Autodesk Fusion 360 part; units mm, degrees
sketch "Sketch1" plane through (0, 0, 0) normal (0, 0, 1) x (1, 0, 0)
  line L0 (75, -95) -> (-75, -95)
  line L1 (-75, -95) -> (-75, 95)
  line L2 (-75, 95) -> (75, 95)
  line L3 (75, 95) -> (75, -95)
  line L4 (75, -95) -> (-75, 95) construction
  line L5 (-75, -95) -> (75, 95) construction
  dimension "d1" = 150
  dimension "d2" = 190
ref_plane "WorkPlane1" through (0, 0, 45) normal (0, 0, 1) x (1, 0, 0)
sketch "Sketch2" plane through (0, 0, 45) normal (0, 0, 1) x (1, 0, 0)
  line L0 (75, -95) -> (-75, -95)
  line L1 (-75, -95) -> (-75, 95)
  line L2 (-75, 95) -> (75, 95)
  line L3 (75, 95) -> (75, -95)
  line L4 (75, -95) -> (-75, 95) construction
  line L5 (-75, -95) -> (75, 95) construction
  dimension "d4" = 150
  dimension "d5" = 190
sketch "Sketch3" plane through (0, 0, 45) normal (0, 0, 1) x (1, 0, 0)
ref_plane "WorkPlane2" through (75, 95, 45) normal (-1, 0, 0) x (0, -1, 0)
sketch "Sketch4" plane through (75, 95, 45) normal (-1, 0, 0) x (0, -1, 0)
  circle A0 centre (155, -22.5) radius 50
  line L0 (0, 0) -> (190, 0)
  circle A1 centre (35, -22.5) radius 50
  dimension "d6" = 100
  dimension "d7" = 22.5
  dimension "d8" = 100
  dimension "d9" = 22.5
  dimension "d10" = 120
  dimension "d11" = 155
ref_plane "WorkPlane3" through (-75, -95, 45) normal (1, 0, 0) x (0, 1, 0)
sketch "Sketch5" plane through (-75, -95, 45) normal (1, 0, 0) x (0, 1, 0)
  circle A0 centre (155, -22.5) radius 50
  circle A1 centre (35, -22.5) radius 50
  line L0 (0, 0) -> (190, 0)
  dimension "d12" = 100
  dimension "d13" = 100
  dimension "d14" = 120
  dimension "d15" = 155
  dimension "d16" = 22.5
  dimension "d17" = 22.5
extrude "Extrude1" add sketch "Sketch2" against normal blind 3 makes body 1
extrude "Extrude2" add sketch "Sketch1" along normal blind 3 separate body makes body 2
extrude "Extrude3" add sketch "Sketch4" against normal blind 40 bodies 1 2
extrude "Extrude4" add sketch "Sketch5" against normal blind 40 bodies 1
sketch "Sketch6" plane through (115, 0, 0) normal (1, 0, 0) x (0, 1, 0)
  circle A0 centre (-60, 22.5) radius 50
  circle A1 centre (-60, 22.5) radius 40
  dimension "d26" = -10
sketch "Sketch7" plane through (115, 0, 0) normal (1, 0, 0) x (0, 1, 0)
  circle A0 centre (60, 22.5) radius 50
  circle A1 centre (60, 22.5) radius 40
  dimension "d27" = -10
extrude "Extrude5" cut sketch "Sketch6" sketch "Sketch7" against normal blind 30 contours A1 of sketch 2 contours A1 bodies 1
sketch "Sketch8" plane through (-115, 0, 0) normal (-1, 0, 0) x (0, -1, 0)
  circle A0 centre (-60, 22.5) radius 50
  circle A1 centre (-60, 22.5) radius 40
  dimension "d30" = -10
sketch "Sketch9" plane through (-115, 0, 0) normal (-1, 0, 0) x (0, -1, 0)
  circle A0 centre (60, 22.5) radius 50
  circle A1 centre (60, 22.5) radius 40
  dimension "d31" = -10
extrude "Extrude6" cut sketch "Sketch8" sketch "Sketch9" against normal blind 30 contours A1 of sketch 2 contours A1 bodies 1
CAD build for the part. Positions are in the model's coordinates, mm. A direction names the side the tool comes from. Coordinates: 2 decimals unless noted, no trailing zeros. Loops run counter-clockwise (first coordinate to the right, second up) from the corner with the lowest first, then second, coordinate; pieces in that order, holes last. Notation, with made-up numbers: (0.5, 2.5) -> (50.5, 2.5) arc R37 cw to (50.5, 39.5) -> close; hole circle Ø8 at (-30.5, -38). An arc over 180 degrees is marked (long way). One line per item, written item: value.
1. Pull direction X, two halves, no side cores. Call faces 6 (the face through (-75, 59, 23)), 7 (the face through (-115, 37.5, 56.1)), 8 (the face through (85, 59, 23)), 9 (the face through (-100.21, -98.153, 34.515)): pulls with the +X half, pulls with the -X half, needs draft (parallel to the pull), parting line crosses it, or undercut.
Answers:
face 6: undercut
face 7: pulls with the -X half
face 8: pulls with the +X half
face 9: needs draft
2. Slice it at B-B on y = 60. Write the cut outline in (x, z), and give its area (3 significant figures).
Answers:
outline: (-115, -27.5) -> (-75, -27.5) -> (-75, 0) -> (75, 0) -> (75, -27.5) -> (115, -27.5) -> (115, -17.5) -> (85, -17.5) -> (85, 62.5) -> (115, 62.5) -> (115, 72.5) -> (75, 72.5) -> (75, 45) -> (-75, 45) -> (-75, 72.5) -> (-115, 72.5) -> (-115, 62.5) -> (-85, 62.5) -> (-85, -17.5) -> (-115, -17.5) -> close; hole (-75, 3) -> (75, 3) -> (75, 42) -> (-75, 42) -> close
area: 4,100 mm^2
3. Flat gauge pins, fed straight in: P1, Ø1, axis at x = 92, z = 31.5, coming from the -Y side; P2, Ø10, axis at x = 65.5, z = 31.5, coming from the +Y side; P3, Ø10, axis at x = -41.5, y = 2.5, coming from the +Z side; P4, Ø3.5, axis at y = 2, z = 1, coming from the -X side. Where does each tip first touch, or does it go through?
Answers:
P1: stops at y = -109.27
P2: passes through
P3: stops at z = 45
P4: stops at x = -75
4. Slice it at C-C on x = 70. Write the cut outline in (y, z).
Answers:
outline: (-95, 0) -> (95, 0) -> (95, 3) -> (-95, 3) -> close; (-95, 42) -> (95, 42) -> (95, 45) -> (-95, 45) -> close
5. Slice it at D-D on y = -6. Write the cut outline in (x, z), and give its area (3 significant figures).
Answers:
outline: (-75, 0) -> (75, 0) -> (75, 3) -> (-75, 3) -> close; (-75, 42) -> (75, 42) -> (75, 45) -> (-75, 45) -> close
area: 900 mm^2
6. Drill centre lines: line 1 (Y direction, x = -94, z = 22); line 2 (Z direction, x = 43.5, y = 3); line 3 (X direction, y = -94.5, z = 48). Where is each one in solid material? Low to high. Write a range as [from, to].
Answers:
line 1: y = [-110, -100], [-20, -10], [10, 20], [100, 110]
line 2: z = [0, 3], [42, 45]
line 3: x = [-115, -75], [75, 115]
7. Which spindle directions (+Z, -Z, +X, -X, +Y, -Y) get a long thin tool onto all of the face, cutting with end or side? Do faces 1 (the face through (-85, -59, 23)), 2 (the face through (-1, 1, 0)), 3 (the face through (-1, 1, 42)), 4 (the face through (115, -37.5, 56.1)), 5 (the face through (-1, 1, 45)). Say none if no direction does.
Answers:
face 1: -X
face 2: -Z, +Y, -Y
face 3: +Y, -Y
face 4: +Z, -Z, +X, +Y, -Y
face 5: +Z, +Y, -Y
8. Slice it at A-A on x = -89. Write the cut outline in (y, z), and give its area (3 significant figures).
Answers:
outline: circle Ø100 at (-60, 22.5); circle Ø100 at (60, 22.5); hole circle Ø80 at (-60, 22.5); hole circle Ø80 at (60, 22.5)
area: 5,650 mm^2
